```python
from build123d import *

# Parameters (mm, degrees)
BOSS_EXTRUDE1_DEPTH       = 2
SKETCH2_W                 = 37
SKETCH2_H                 = 2
SKETCH2_H_2               = 2.001734714
BOSS_EXTRUDE2_DEPTH       = 8
FILLET1_R                 = 2
FILLET2_R                 = 0.25
TAP_DRILL_FOR_M2_5_TAP1_D = 2.05
SKETCH5_R                 = 5
CUT_EXTRUDE1_DEPTH        = 28.699277969
M2_5_CLEARANCE_HOLE1_D    = 2.9
CIRPATTERN1_COUNT         = 8
M2_5_CLEARANCE_HOLE2_D    = 2.9


with BuildPart() as part:
    # Sketch1 → Boss-Extrude1 (new body)
    with BuildSketch(Plane(origin=(0, 0, 0), x_dir=(1, 0, 0), z_dir=(0, 1, 0))):
        with BuildLine():
            Line((-14.5, 3), (-18.5, 3))
            Line((-18.5, 3), (-18.5, 19))
            Line((-18.5, 19), (18.5, 19))
            Line((18.5, 19), (18.5, -19))
            Line((18.5, -19), (-18.5, -19))
            Line((-18.5, -19), (-18.5, -3))
            Line((-18.5, -3), (-14.5, -3))
            ThreePointArc((-14.5, -3), (-11.5, 0), (-14.5, 3))
        make_face()
    extrude(amount=BOSS_EXTRUDE1_DEPTH)

    # Sketch2 → Boss-Extrude2 (add)
    with BuildSketch(Plane(origin=(0, 2, 0), x_dir=(1, 0, 0), z_dir=(0, 1, 0))):
        with Locations((0, 18)):
            Rectangle(SKETCH2_W, SKETCH2_H)
        with Locations((0, -17.999132643)):
            Rectangle(SKETCH2_W, SKETCH2_H_2)
    extrude(amount=BOSS_EXTRUDE2_DEPTH)

    # Fillet1
    fillet1_edges = [part.edges().sort_by_distance(p)[0] for p in [
        (0, 0, -19),
        (-18.5, 10, -18),
        (18.5, 10, -18),
        (-18.5, 10, 17.999132643),
        (18.5, 10, 17.999132643),
        (0, 0, 19),
    ]]
    fillet(fillet1_edges, radius=FILLET1_R)

    # Fillet2
    fillet2_edges = [part.edges().sort_by_distance(p)[0] for p in [
        (0, 2, -17),
        (0, 2, 16.998265286),
    ]]
    fillet(fillet2_edges, radius=FILLET2_R)

    # Tap Drill for M2.5 Tap1 (through all)
    with Locations(Plane(origin=(0, 2, 0), x_dir=(1, 0, 0), z_dir=(0, 1, 0))):
        with Locations((-13.5, 13), (14.5, 13), (14.5, -13), (-13.5, -13)):
            Hole(TAP_DRILL_FOR_M2_5_TAP1_D / 2)

    # Sketch5 → Cut-Extrude1 (cut, through all)
    with BuildSketch(Plane(origin=(0, 2, 0), x_dir=(1, 0, 0), z_dir=(0, 1, 0))):
        with Locations(Location((3.5, 0, 0), (0, 0, 270))):
            Circle(SKETCH5_R)
    extrude(amount=-CUT_EXTRUDE1_DEPTH, mode=Mode.SUBTRACT)

    # M2.5 Clearance Hole1 (through all)
    with Locations(Plane(origin=(0, 2, 0), x_dir=(1, 0, 0), z_dir=(0, 1, 0))):
        with Locations((3.5, 11)):
            m2_5_clearance_hole1 = Hole(M2_5_CLEARANCE_HOLE1_D / 2)

    # CirPattern1: M2.5 Clearance Hole1 ×8 about axis
    cirpattern1_axis = Axis((3.5, 0, 0), (0, 1, 0))
    for i in range(1, CIRPATTERN1_COUNT):
        add(m2_5_clearance_hole1.rotate(cirpattern1_axis, i * 360 / CIRPATTERN1_COUNT), mode=Mode.SUBTRACT)

    # M2.5 Clearance Hole2 (through all)
    with Locations(Plane.XY.offset(19)):
        with Locations((-14.5, 5.870134778), (-7.5, 5.870134778), (7.5, 5.870134778), (14.5, 5.870134778)):
            Hole(M2_5_CLEARANCE_HOLE2_D / 2)


solid = part.part
```
CAD build for the part. Positions are in the model's coordinates, mm. A direction names the side the tool comes from. Coordinates: 2 decimals unless noted, no trailing zeros. Order: outer loops, then holes, each group sorted by start corner. A loop starts at its lowest first (then second) coordinate and runs counter-clockwise, first axis right, second up.
(1) Mould opens along X. For faces 1 (the face through (-18.5, 1.6, -12.1)), 2 (the face through (-0.26, 0.6, 18.43)), 3 (the face through (-4.592, 0.986, 9.194)) say: released by +X, released by -X, zero draft, split by the parting line, or undercut.
Solution:
face 1: released by -X
face 2: zero draft
face 3: undercut
(2) Saw through at A-A, the plane x = -7.5. Write the cut outline in (y, z).
Solution:
outline: (0, -17) arc R2 ccw to (2, -19) - (4.42, -19) - (4.42, -17) - (2.25, -17) arc R0.25 cw to (2, -16.75) - (2, -1.45) - (0, -1.45) - close; (0, 1.45) - (2, 1.45) - (2, 16.75) arc R0.25 cw to (2.25, 17) - (4.42, 17) - (4.42, 19) - (2, 19) arc R2 ccw to (0, 17) - close; (7.32, -19) - (10, -19) - (10, -17) - (7.32, -17) - close; (7.32, 17) - (10, 17) - (10, 19) - (7.32, 19) - close
(3) Pin check, flat tips, straight feed: pin 1 Ø1.6 at (x, z) = (14.5, 13) entering from +Y; pin 2 Ø10 at (x, z) = (7, 6) entering from +Y. Stop position of each tip, or through.
Solution:
pin 1: passes through
pin 2: stops at y = 2
(4) Saw through at B-B, the plane z = -13. Write the cut outline in (x, y) (3 decimals).
Solution:
outline: (-18.5, 0) - (-14.525, 0) - (-14.525, 2) - (-18.5, 2) - close; (-12.475, 0) - (13.475, 0) - (13.475, 2) - (-12.475, 2) - close; (15.525, 0) - (18.5, 0) - (18.5, 2) - (15.525, 2) - close
(5) Saw through at D-D, the plane y = 3.5. Write the cut outline in (x, z).
Solution:
outline: (-18.5, -19) - (18.5, -19) - (18.5, -17) - (-18.5, -17) - close; (-18.5, 17) - (18.5, 17) - (18.5, 19) - (-18.5, 19) - close
(6) Which spindle directions (+Z, -Z, +X, -X, +Y, -Y) get a long thin tool onto all of the face, cutting with end or side? Do faces 4 (the face through (-18.5, 1.6, 12.2)), 5 (the face through (0, 6, 16.998)), 6 (the face through (-17, 1, 3)). Say none if no direction does.
Solution:
face 4: +Z, -Z, -X, +Y, -Y
face 5: +X, -X, +Y
face 6: -X, +Y, -Y
(7) Saw through at C-C, the plane z = 4. Write the cut outline in (x, y).
Solution:
outline: (-18.5, 0) - (0.5, 0) - (0.5, 2) - (-18.5, 2) - close; (6.5, 0) - (18.5, 0) - (18.5, 2) - (6.5, 2) - close
(8) Drill centre lines: L1, parallel to X at y = 0.5, z = -13 (3 decimals); L2, parallel to Z at x = 4, y = 7.75; L3, parallel to Z at x = -13.5, y = 0.8 (3 decimals). Where is each one in solid material? Low to high.
Solution:
L1: x = -18.5 to -14.525, -12.475 to 13.475, 15.525 to 18.5
L2: z = -19 to -17, 17 to 19
L3: z = -18.6 to -14.025, -11.975 to -2.828, 2.828 to 11.975, 14.025 to 18.6
